Source: CAD feature listing. Evaluate the final solid. Frame: model axes, mm. Round coordinates to 2 decimals unless told otherwise and drop trailing zeros. Order: outer loops, then holes, each group sorted by start corner. A loop starts at its lowest first (then second) coordinate and runs counter-clockwise, first axis right, second up. Notation, with made-up numbers: M 47,40 L 71,40 A31 cw 71,69 Z; hole C -35,27.25 d2. An arc over 180 degrees is marked long. Use one line per item in the form item = value. Start each with the question number.
Q1. Material intervals for probe 1 along Y at (x, z) = (0, 4.7); probe 2 along Y at (x, z) = (78, 4.25); probe 3 along X at (y, z) = (-7.5, 4.9), sorted ascending.
Q2. Section B-B (y = 0). Return the cut outline in (x, z), plus the area to 3 significant figures.
Q3. Contact query for flat-ended pins moving along their axis: pin 1 (3 mm diameter, centred on y = -21, z = 4, fed in from +X); pin 2 (1 mm diameter, centred on x = -5.5, z = 4, fed in from +Y). Output: stop coordinate, or through.
Q4. Section C-C (z = 1.7). Return the cut outline in (x, y), plus the area to 3 significant figures.
Q5. Section A-A (x = 0). Return the cut outline in (y, z).
Q6. Pull-direction query (X, two-part tool) for faces 1 (the flat face through (23, 1, 6)), 2 (the flat face through (51.292, 26.173, 2.958)), 3 (the cylindrical face through (23.772, -22.15, 3.042)); classes: pulls with the +X half, pulls with the -X half, needs draft (parallel to the pull), parting line crosses it, or undercut.
Q7. Section D-D (x = 80). Return the cut outline in (y, z), plus the area to 3 significant figures.
from build123d import *

# Parameters (mm, degrees)
SKETCH_R     = 14.3
SKETCH_R_2   = 3.1
PAD_DEPTH    = 6
SKETCH001_R  = 3
POCKET_DEPTH = 10


with BuildPart() as part:
    # Sketch → Pad (new body)
    with BuildSketch(Plane.XY):
        with BuildLine():
            ThreePointArc((18.562462, 40.993109), (-45, 0), (18.562462, -40.993109))
            Line((18.562462, -40.993109), (84.949967, -10.931506))
            ThreePointArc((84.949967, -10.931506), (92, 0), (84.949967, 10.931506))
            Line((18.562462, 40.993109), (84.949967, 10.931506))
        make_face()
        Circle(SKETCH_R, mode=Mode.SUBTRACT)
        with Locations((80, 0)):
            Circle(SKETCH_R_2, mode=Mode.SUBTRACT)
    extrude(amount=PAD_DEPTH)

    # Sketch001 → Pocket (cut)
    with BuildSketch(Plane.XY.offset(6)):
        with Locations((-21.001071, 21.001071)):
            Circle(SKETCH001_R)
        with Locations((21.001071, 21.001071)):
            Circle(SKETCH001_R)
        with Locations((-21.001071, -21.001071)):
            Circle(SKETCH001_R)
        with Locations((21.001071, -21.001071)):
            Circle(SKETCH001_R)
    extrude(amount=-POCKET_DEPTH, mode=Mode.SUBTRACT)


solid = part.part
Results list:
q1.probe_1 = -45 to -14.3, 14.3 to 45
q1.probe_2 = -14.08 to -2.37, 2.37 to 14.08
q1.probe_3 = -44.37 to -12.18, 12.18 to 89.37
q2.outline = M -45,0 L -14.3,0 L -14.3,6 L -45,6 Z; M 14.3,0 L 76.9,0 L 76.9,6 L 14.3,6 Z; M 83.1,0 L 92,0 L 92,6 L 83.1,6 Z
q2.area = 613 mm2
q3.pin_1 = 66.03
q3.pin_2 = 44.72
q4.outline = M 18.56,-40.99 L 84.95,-10.93 A12 ccw 84.95,10.93 L 18.56,40.99 A45 ccw long Z; hole C -21,-21 d6; hole C -21,21 d6; hole C 0,0 d28.6; hole C 21,-21 d6; hole C 21,21 d6; hole C 80,0 d6.2
q4.area = 7,580 mm2
q5.outline = M -45,0 L -14.3,0 L -14.3,6 L -45,6 Z; M 14.3,0 L 45,0 L 45,6 L 14.3,6 Z
q6.face_1 = needs draft
q6.face_2 = pulls with the +X half
q6.face_3 = undercut
q7.outline = M -13.17,0 L -3.1,0 L -3.1,6 L -13.17,6 Z; M 3.1,0 L 13.17,0 L 13.17,6 L 3.1,6 Z
q7.area = 121 mm2
